Part model, mm, in its own coordinate system. A direction names the side the tool comes from. Coordinates: 2 decimals unless noted, no trailing zeros. Loops run counter-clockwise (first coordinate to the right, second up) from the corner with the lowest first, then second, coordinate; pieces in that order, holes last. Notation, with made-up numbers: (55.25, 14.5) - (94.25, 14.5) arc R28 cw to (94.25, 48.5) - close; hole circle Ø1 at (-2, -29). An arc over 180 degrees is marked (long way). Answer as CSV lines item,"result".
from build123d import *

# Parameters (mm, degrees)
SKETCH_W        = 51.5
SKETCH_H        = 48
PAD_DEPTH       = 10
SKETCH001_R     = 1.6
POCKET_DEPTH    = 51.501
FILLET_R        = 3
PAD001_DEPTH    = 48
SKETCH003_R     = 1.8
POCKET001_DEPTH = 11.561
SKETCH004_R     = 2.8
POCKET002_DEPTH = 3
SKETCH005_W     = 9.48
SKETCH005_H     = 9.48
POCKET003_DEPTH = 1.56
POCKET004_DEPTH = 10.001


with BuildPart() as part:
    # Sketch → Pad (new body)
    with BuildSketch(Plane.XY):
        Rectangle(SKETCH_W, SKETCH_H)
    extrude(amount=PAD_DEPTH)

    # Sketch001 (on Face4 of Pad) → Pocket (cut, through all)
    with BuildSketch(Plane(origin=(-25.75, 0, 0), x_dir=(0, -1, 0), z_dir=(-1, 0, 0))):
        with Locations((-15.8, 5)):
            Circle(SKETCH001_R)
        with Locations((15.8, 5)):
            Circle(SKETCH001_R)
    extrude(amount=-POCKET_DEPTH, mode=Mode.SUBTRACT)

    # Fillet
    fillet_edges = [part.edges().sort_by_distance(p)[0] for p in [
        (25.75, -24, 5),
        (25.75, 24, 5),
        (-25.75, 24, 5),
        (-25.75, -24, 5),
    ]]
    fillet(fillet_edges, radius=FILLET_R)

    # Sketch002 (on Face1 of Fillet) → Pad001 (join)
    with BuildSketch(Plane(origin=(0, 24, 0), x_dir=(-1, 0, 0), z_dir=(0, 1, 0))):
        Polygon((2.94, 11.56), (-2.94, 11.56), (-4.74, 10), (4.74, 10), align=None)
    extrude(amount=-PAD001_DEPTH)

    # Sketch003 (on Face14 of Pad001) → Pocket001 (cut, through all)
    with BuildSketch(Plane.XY.offset(11.56)):
        with Locations((0, 10)):
            Circle(SKETCH003_R)
        with Locations((0, -10)):
            Circle(SKETCH003_R)
    extrude(amount=-POCKET001_DEPTH, mode=Mode.SUBTRACT)

    # Sketch004 (on Face2 of Pocket001) → Pocket002 (cut)
    with BuildSketch(Plane(origin=(0, 0, 0), x_dir=(1, 0, 0), z_dir=(0, 0, -1))):
        with Locations((0, 10)):
            Circle(SKETCH004_R)
        with Locations((0, -10)):
            Circle(SKETCH004_R)
    extrude(amount=-POCKET002_DEPTH, mode=Mode.SUBTRACT)

    # Sketch005 (on Face16 of Pocket002) → Pocket003 (cut)
    with BuildSketch(Plane.XY.offset(11.56)):
        with Locations((0, 10)):
            Rectangle(SKETCH005_W, SKETCH005_H)
        with Locations((0, -10)):
            Rectangle(SKETCH005_W, SKETCH005_H)
    extrude(amount=-POCKET003_DEPTH, mode=Mode.SUBTRACT)

    # Sketch006 (on Face5 of Pocket003) → Pocket004 (cut, through all)
    with BuildSketch(Plane.XY.offset(10)):
        with BuildLine():
            ThreePointArc((-9.74, 13.495), (-15.245, 19), (-20.75, 13.495))
            Line((-20.75, 13.495), (-20.75, -13.495))
            ThreePointArc((-20.75, -13.495), (-15.245, -19), (-9.74, -13.495))
            Line((-9.74, -13.495), (-9.74, 13.495))
        make_face()
        with BuildLine():
            ThreePointArc((20.75, 13.495), (15.245, 19), (9.74, 13.495))
            Line((9.74, 13.495), (9.74, -13.495))
            ThreePointArc((9.74, -13.495), (15.245, -19), (20.75, -13.495))
            Line((20.75, -13.495), (20.75, 13.495))
        make_face()
    extrude(amount=-POCKET004_DEPTH, mode=Mode.SUBTRACT)


solid = part.part
Q1. Wall check: L1, parallel to Y at x = 0, z = 1; L2, parallel to X at y = -1, z = 5.5; L3, parallel to Y at x = 22.5, z = 5. Give the ranges that are in metal, low to high.
Results:
L1,"y = -24 to -12.8, -7.2 to 7.2, 12.8 to 24"
L2,"x = -25.75 to -20.75, -9.74 to 9.74, 20.75 to 25.75"
L3,"y = -24 to -17.4, -14.2 to 14.2, 17.4 to 24"
Q2. Saw through at A-A (x = 0). Count the separate pieces of the cut face and the enclosed holes in it, then the cut area to 3 significant figures.
Results:
separate pieces,"3"
enclosed holes,"2"
area,"425 mm^2"
Q3. Saw through at D-D (y = 6). Give the cut face in (x, z), then the cut area to 3 significant figures.
Results:
outline,"(-25.75, 0) - (-20.75, 0) - (-20.75, 10) - (-25.75, 10) - close; (-9.74, 0) - (9.74, 0) - (9.74, 10) - (-9.74, 10) - close; (20.75, 0) - (25.75, 0) - (25.75, 10) - (20.75, 10) - close"
area,"295 mm^2"
Q4. Two-plate mould, pull along Y, no slides. Class faces 1 (the face through (-3.85, 0.07, 10.77)), 2 (the face through (-0.607, 12.733, 1.479)), 3 (the face through (24.85, -23.14, 5.07)): released by +Y, released by -Y, zero draft, split by the parting line, or undercut.
Results:
face 1,"zero draft"
face 2,"undercut"
face 3,"released by -Y"
Q5. Saw through at C-C (z = 8.25). Give the cut face in (x, y) (3 decimals).
Results:
outline,"(-25.75, -21) arc R3 ccw to (-22.75, -24) - (22.75, -24) arc R3 ccw to (25.75, -21) - (25.75, 21) arc R3 ccw to (22.75, 24) - (-22.75, 24) arc R3 ccw to (-25.75, 21) - close; hole (-20.75, -13.495) arc R5.505 ccw to (-9.74, -13.495) - (-9.74, 13.495) arc R5.505 ccw to (-20.75, 13.495) - close; hole circle Ø3.6 at (0, -10); hole circle Ø3.6 at (0, 10); hole (9.74, -13.495) arc R5.505 ccw to (20.75, -13.495) - (20.75, 13.495) arc R5.505 ccw to (9.74, 13.495) - close"
Q6. Saw through at B-B (y = -10). Give the cut face in (x, z), then the cut area to 3 significant figures.
Results:
outline,"(-25.75, 0) - (-20.75, 0) - (-20.75, 10) - (-25.75, 10) - close; (-9.74, 0) - (-2.8, 0) - (-2.8, 3) - (-1.8, 3) - (-1.8, 10) - (-9.74, 10) - close; (1.8, 3) - (2.8, 3) - (2.8, 0) - (9.74, 0) - (9.74, 10) - (1.8, 10) - close; (20.75, 0) - (25.75, 0) - (25.75, 10) - (20.75, 10) - close"
area,"253 mm^2"
Q7. Which spindle directions (+Z, -Z, +X, -X, +Y, -Y) get a long thin tool onto all of the face, cutting with end or side? Do faces 4 (the face through (-25.75, 0, 5)), 5 (the face through (9.74, 0, 5)). Say none if no direction does.
Results:
face 4,"+Z, -Z, -X, +Y, -Y"
face 5,"+Z, -Z"
Q8. Flat gauge pins, fed straight in: pin 1 (1.7 mm diameter, centred on x = -1.5, y = 10, fed in from -Z); pin 2 (6 mm diameter, centred on x = 0, y = 10, fed in from +Z). Where does each tip first touch, or does it go through?
Results:
pin 1,"stops at z = 3"
pin 2,"stops at z = 10"
